Autodesk Inventor part; units mm, degrees
ref_plane "YZ Plane" through (0, 0, 0) normal (1, 0, 0) x (0, 1, 0)
ref_plane "XZ Plane" through (0, 0, 0) normal (0, 1, 0) x (-1, 0, 0)
ref_plane "XY Plane" through (0, 0, 0) normal (0, 0, 1) x (1, 0, 0)
sketch "Sketch1" plane through (0, 0, 0) normal (0, 1, 0) x (-1, 0, 0)
  line L0 (-107.95, 57.5) -> (107.95, 57.5)
  line L1 (107.95, 57.5) -> (107.95, -57.5)
  line L2 (107.95, -57.5) -> (-107.95, -57.5)
  line L3 (-107.95, -57.5) -> (-107.95, 57.5)
  line L4 (-107.95, 57.5) -> (107.95, -57.5) construction
  line L5 (107.95, 57.5) -> (-107.95, -57.5) construction
  point P0 (0, 0)
  dimension "d0" = 215.9
  dimension "d1" = 115
extrude "Extrusion1" add sketch "Sketch1" along normal blind 30
sketch "Sketch2" plane through (0, 30, 0) normal (0, 1, 0) x (1, 0, 0)
  line L0 (107.95, 57.5) -> (-107.95, 57.5)
  line L1 (-107.95, 57.5) -> (-107.95, -57.5)
  line L2 (-107.95, -57.5) -> (107.95, -57.5)
  line L3 (107.95, -57.5) -> (107.95, 57.5)
  line L4 (-91.95, 57.5) -> (-91.95, -57.5)
  point P0 (0, 0)
  dimension "d4" = 16
extrude "Extrusion2" cut sketch "Sketch2" against normal blind 25 contours L4 L2 L1 L0
sketch "Sketch3" plane through (0, 0, 0) normal (0, -1, 0) x (1, 0, 0)
  line L0 (-74.05, 25) -> (75.95, 25) construction
  line L1 (75.95, 25) -> (75.95, -25) construction
  line L2 (107.95, 57.5) -> (107.95, -57.5) construction
  line L3 (0, 0) -> (75.95, 0) construction
  circle A0 centre (-74.05, 25) radius 2
  circle A1 centre (75.95, 25) radius 2
  circle A2 centre (75.95, -25) radius 2
  line L4 (-74.05, 25) -> (-74.05, -25) construction
  circle A3 centre (-74.05, -25) radius 2
  line L5 (107.95, -57.5) -> (-107.95, -57.5) construction
  line L6 (107.95, 57.5) -> (107.95, -57.5)
  line L7 (-107.95, 57.5) -> (107.95, 57.5) construction
  line L8 (-107.95, -57.5) -> (-107.95, 57.5) construction
  dimension "d7" = 150
  dimension "d8" = 50
  dimension "d9" = 32
  dimension "d10" = 4
extrude "Extrusion3" cut sketch "Sketch3" against normal blind 4
properties part number "Stepper Power Supply"
Could you check a few things on this model? Use its own coordinates, in mm. A direction names the side the tool comes from. Give positions to 0.01 mm unless a question says otherwise; leave off trailing zeros. Order: outer loops, then holes, each group sorted by start corner. A loop starts at its lowest first (then second) coordinate and runs counter-clockwise, first axis right, second up.
Q1. We'd pull the mould along Z, two halves only. Please class faces 4 (the flat face through (9, 30, 1)), 5 (the flat face through (2, 15, 57.5)), 6 (the flat face through (76, 4, -25)): +Z half, -Z half, draft (parallel to the pull), parting line (faces both ways), or undercut.
Q2. I'm going to push flat-ended pins straight in: P1, Ø1.2, axis at x = 76, z = 25.5, coming from the -Y side; P2, Ø3, axis at y = 10, z = -9, coming from the -X side. Where does each tip first touch, or does it pass through?
Q3. Suppose I cut it at B-B, the plane y = 19.25. Write out the boundary of the cut face in (x, z).
Q4. For faces 1 (the flat face through (-100, 5, -1)), 2 (the flat face through (76, 4, 25)), 3 (the flat face through (-2, 15, -57.5)), which set-ups out of +Z, -Z, +X, -X, +Y, -Y let a thin tool reach every point of the face, with its end or its side?
Q5. If I drill on line 1 along Z through (x, y) = (75.95, 1); line 2 along Y through (x, z) = (-96, 42.5); line 3 along X through (y, z) = (20.75, -3), over which ranges is the centre line in solid material (lowest first)?
Q6. Suppose I cut it at A-A, the plane z = -25. Write out the boundary of the cut face in (x, y), and give its area (4 significant figures).
Solution:
1. face 4: draft
1. face 5: +Z half
1. face 6: undercut
2. P1: stops at y = 4
2. P2: stops at x = -91.95
3. outline: (-91.95, -57.5) - (107.95, -57.5) - (107.95, 57.5) - (-91.95, 57.5) - close
4. face 1: +Z, -Z, -X, +Y
4. face 2: -Y
4. face 3: -Z, +X, -X, +Y, -Y
5. line 1: z = -57.5 to -27, -23 to 23, 27 to 57.5
5. line 2: y = 0 to 5
5. line 3: x = -91.95 to 107.95
6. outline: (-107.95, 0) - (-76.05, 0) - (-76.05, 4) - (-72.05, 4) - (-72.05, 0) - (73.95, 0) - (73.95, 4) - (77.95, 4) - (77.95, 0) - (107.95, 0) - (107.95, 30) - (-91.95, 30) - (-91.95, 5) - (-107.95, 5) - close
6. area: 6,045 mm2
